The model under review builds one solid part; all positions refer to its coordinate system, in mm. Face numbers are marked on the shaded views. A direction names the side the tool comes from. Coordinates: 2 decimals unless noted, no trailing zeros. Write each loop counter-clockwise with the first axis right and the second up, starting at its lowest first coordinate (ties: lowest second). Pieces come first, ordered by that corner, then holes. Notation, with made-up numbers: M 17,-11.75 L 74,-11.75 A31 cw 74,19.25 Z; hole C -6,-9 d7. An arc over 180 degrees is marked long. Answer as a JSON object with one key per item and string values.
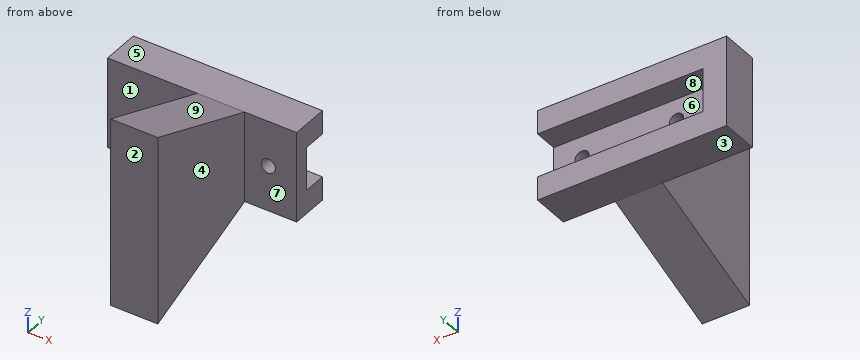
```python
from build123d import *

# Parameters (mm, degrees)
BOSS_EXTRUDE1_DEPTH      = 26
BOSS_EXTRUDE1_DEPTH_BACK = 9
CUT_EXTRUDE1_DEPTH       = 29.163096421
CUT_EXTRUDE1_DEPTH_BACK  = 29.163096421
SKETCH4_R                = 1.5
BOSS_EXTRUDE2_DEPTH      = 5
SKETCH7_W                = 19.2
SKETCH7_H                = 8
BOSS_EXTRUDE3_DEPTH      = 5


with BuildPart() as part:
    # Sketch3 → Boss-Extrude1 (new, two sides: drawn at the far end of the back side and taken through both)
    with BuildSketch(Plane(origin=(0, 0, 0), x_dir=(0, 0, -1), z_dir=(1, 0, 0)).offset(-BOSS_EXTRUDE1_DEPTH_BACK)):
        Polygon((-4.6, 0), (-4.6, 5), (-9.6, 5), (-9.6, -3), (9.6, -3), (9.6, 5), (4.6, 5), (4.6, 0), align=None)
    extrude(amount=BOSS_EXTRUDE1_DEPTH + BOSS_EXTRUDE1_DEPTH_BACK)

    # Sketch4 → Cut-Extrude1 (cut, two sides: drawn at the far end of the back side and taken through both)
    with BuildSketch(Plane(origin=(0, 0, 0), x_dir=(1, 0, 0), z_dir=(0, 1, 0)).offset(-CUT_EXTRUDE1_DEPTH_BACK)):
        with Locations(Location((0, 0, 0), (0, 0, 270))):
            Circle(SKETCH4_R)
        with Locations(Location((20, 0, 0), (0, 0, 270))):
            Circle(SKETCH4_R)
    extrude(amount=CUT_EXTRUDE1_DEPTH + CUT_EXTRUDE1_DEPTH_BACK, mode=Mode.SUBTRACT)

    # Sketch6 → Boss-Extrude2 (add, symmetric)
    with BuildSketch(Plane(origin=(10, 0, 0), x_dir=(0, 0, -1), z_dir=(1, 0, 0))):
        Polygon((-20, -30), (-9.6, -3), (9.6, -3), (20, -30), align=None)
    extrude(amount=BOSS_EXTRUDE2_DEPTH, both=True)

    # Sketch7 → Boss-Extrude3 (add)
    with BuildSketch(Plane.ZY.offset(9)):
        with Locations((0, 1)):
            Rectangle(SKETCH7_W, SKETCH7_H)
    extrude(amount=BOSS_EXTRUDE3_DEPTH)


solid = part.part
```
(1) For pin 1 Ø1 at (x, y) = (10, -11.5) entering from -Z; pin 2 Ø3.5 at (x, z) = (22, -2) entering from -Y; pin 3 Ø1 at (y, z) = (-23, -3) entering from +X; pin 4 Ø1.8 at (x, z) = (20, 0) entering from +Y, all flat-tipped, find the tip position at first contact; note any pin that passes through.
Results list:
{"pin 1": "z = -13.07", "pin 2": "y = -3", "pin 3": "x = 15", "pin 4": "through"}
(2) Draft analysis for pull direction Z (two halves, no side actions). For the marked faces 6, 7, 8 and 9, state which applies: released by +Z, released by -Z, zero draft, split by the parting line, or undercut.
Results list:
{"face 6": "undercut", "face 7": "zero draft", "face 8": "undercut", "face 9": "released by +Z"}
(3) Add section D-D on x = 6.5. Give the boundary of the cut face in (y, z), and give its area (3 significant figures).
Results list:
{"outline": "M -30,-20 L -3,-9.6 L 5,-9.6 L 5,-4.6 L 0,-4.6 L 0,4.6 L 5,4.6 L 5,9.6 L -3,9.6 L -30,20 Z", "area": "907 mm²"}
(4) For the marked faces 1, 2, 3, 4 and 5, list the 3-axis set-ups (+Z, -Z, +X, -X, +Y, -Y) from which the entire face can be reached by the end or side of a thin tool; tool diameter is ignored.
Results list:
{"face 1": "+Z, -Z, -X, -Y", "face 2": "+Z, -Z, +X, -X, -Y", "face 3": "-Z, +X, -X, +Y", "face 4": "+Z, -Z, +X, -Y", "face 5": "+Z, +X, -X, +Y"}
(5) Add section B-B on x = 20. Give the boundary of the cut face in (y, z).
Results list:
{"outline": "M -3,-9.6 L 5,-9.6 L 5,-4.6 L 0,-4.6 L 0,-1.5 L -3,-1.5 Z; M -3,1.5 L 0,1.5 L 0,4.6 L 5,4.6 L 5,9.6 L -3,9.6 Z"}
(6) Add section A-A on z = 0. Give the boundary of the cut face in (x, y).
Results list:
{"outline": "M -14,-3 L -1.5,-3 L -1.5,0 L -9,0 L -9,5 L -14,5 Z; M 1.5,-3 L 5,-3 L 5,-30 L 15,-30 L 15,-3 L 18.5,-3 L 18.5,0 L 1.5,0 Z; M 21.5,-3 L 26,-3 L 26,0 L 21.5,0 Z"}
(7) Wall thickness on line 1 along X through (y, z) = (-1.3, 0); line 2 along Z through (x, y) = (20, -2); line 3 along Z through (x, y) = (-6, 3): over which ranges is each line inside the solid? List them lowest first. Write a range as from..to.
Results list:
{"line 1": "-14..-1.5, 1.5..18.5, 21.5..26", "line 2": "-9.6..-1.5, 1.5..9.6", "line 3": "-9.6..-4.6, 4.6..9.6"}
(8) Add section C-C on z = -8. Give the boundary of the cut face in (x, y).
Results list:
{"outline": "M -14,-3 L 5,-3 L 5,-30 L 15,-30 L 15,-3 L 26,-3 L 26,5 L -14,5 Z"}
